```python
from build123d import *

# Parameters (mm, degrees)
SKETCH_1_W          = 45
SKETCH_1_H          = 4
SKETCH_1_W_2        = 5
EXTRUDE_1_DEPTH     = 84
SKETCH_2_W          = 20
SKETCH_2_H          = 20
CUT_EXTRUDE_1_DEPTH = 14
EXTRUDE_2_DEPTH     = 84


with BuildPart() as part:
    # Эскиз1 → Бобышка-Вытянуть1 (new body)
    with BuildSketch(Plane(origin=(0, 0, 0), x_dir=(0, 0, -1), z_dir=(1, 0, 0))):
        with Locations((22.5, 2)):
            Rectangle(SKETCH_1_W, SKETCH_1_H)
        with Locations((47.5, 2)):
            Rectangle(SKETCH_1_W_2, SKETCH_1_H)
        Polygon((45, 29), (45, 4), (50, 4), (50, 26.569712745), (48.596872999, 29), align=None)
        with Locations((22.5, 31)):
            Rectangle(SKETCH_1_W, SKETCH_1_H)
        Polygon((45, 33), (45, 29), (48.596872999, 29), (46.287471923, 33), align=None)
        Polygon((48.596872999, 29), (50, 26.569712745), (50, 29), align=None)
        Polygon((50, 29), (50, 26.569712745), (65.186719292, 0.265543331), (68.650820907, 2.265543331), (8.650820907, 106.188591785), (5.186719292, 104.188591785), (46.287471923, 33), (50, 33), align=None)
        Polygon((46.287471923, 33), (48.596872999, 29), (50, 29), (50, 33), align=None)
    extrude(amount=EXTRUDE_1_DEPTH)

    # Эскиз2 → Вырез-Вытянуть1 (cut)
    with BuildSketch(Plane.XZ):
        with Locations((74, -10)):
            Rectangle(SKETCH_2_W, SKETCH_2_H)
    extrude(amount=-CUT_EXTRUDE_1_DEPTH, mode=Mode.SUBTRACT)

    # Эскиз3 → Бобышка-Вытянуть2 (add)
    with BuildSketch(Plane(origin=(84, 0, 0), x_dir=(0, 0, -1), z_dir=(1, 0, 0))):
        Polygon((68.650820907, 2.265543331), (72.114922522, 4.265543331), (70.614922522, 6.863619543), (67.150820907, 4.863619543), align=None)
        Polygon((40.778226629, 42.54229276), (40.778226629, 33), (46.287471923, 33), align=None)
        Polygon((50, 26.569712745), (50, 18.552766001), (54.628586361, 18.552766001), align=None)
    extrude(amount=-EXTRUDE_2_DEPTH)


solid = part.part
```
The model under review builds one solid part; all positions refer to its coordinate system, in mm. A direction names the side the tool comes from. Coordinates: 2 decimals unless noted, no trailing zeros. Write each loop counter-clockwise with the first axis right and the second up, starting at its lowest first coordinate (ties: lowest second). Pieces come first, ordered by that corner, then holes. Notation, with made-up numbers: (7.25, 30) -> (58.25, 30) arc R19 cw to (58.25, 60) -> close; hole circle Ø5 at (82.25, 85). An arc over 180 degrees is marked (long way). One line per item, written item: value. Start each with the question number.
Q1. Add section D-D, the plane y = 27.5. Give the boundary of the cut face in (x, z).
Q2. The part is to be moulded in two halves that separate along Z. For faces 5 (the face through (42.6, 5.5, -71.4)), 6 (the face through (41, 9, -50)), 7 (the face through (64, 2, -10)), say which applies: +Z half, -Z half, draft (parallel to the pull), parting line (faces both ways), or undercut.
Q3. To check wall thickness, follow probe 1 along Y at (x, z) = (54, -4); probe 2 along Y at (x, z) = (61, -33); probe 3 along Y at (x, z) = (76, -23.5). State the ranges of each line that lie inside material, in increasing order.
Q4. Add section A-A, the plane z = -33. Give the boundary of the cut face in (x, y), then the cut area to 3 significant figures.
Q5. Clearance check with flat-ended pins moving along their axes: P1, Ø13.5, axis at x = 46.5, z = -28, coming from the +Y side; P2, Ø2.5, axis at x = 51, z = -52, coming from the -Y side; P3, Ø3, axis at x = 31.5, y = 55, coming from the -Z side; P4, Ø3, axis at x = 62.5, z = -16.5, coming from the -Y side. State where each tip first meets the part, or that it passes through.
Q6. Add section B-B, the plane x = 54. Give the boundary of the cut face in (y, z), then the cut area to 3 significant figures.
Q7. For faces 1 (the face through (74, 2, -20)), 2 (the face through (42.59, 5.88, -68.91)), 3 (the face through (41, 17, -45)), 4 (the face through (41.41, 9.54, -59.83)), list the 3-axis set-ups (+Z, -Z, +X, -X, +Y, -Y) from which the entire face can be reached by the end or side of a thin tool; tool diameter is ignored.
Q8. Add section C-C, the plane x = 67. Give the boundary of the cut face in (y, z), then the cut area to 3 significant figures.
Response:
1. outline: (0, -54.08) -> (84, -54.08) -> (84, -45) -> (0, -45) -> close
2. face 5: -Z half
2. face 6: undercut
2. face 7: draft
3. probe 1: 0 to 4, 29 to 33
3. probe 2: 0 to 4, 29 to 33, 56.01 to 64.01
3. probe 3: 0 to 4, 29 to 33, 72.47 to 80.47
4. outline: (0, 0) -> (84, 0) -> (84, 4) -> (0, 4) -> close; (0, 29) -> (84, 29) -> (84, 33) -> (0, 33) -> close; (0, 56.01) -> (84, 56.01) -> (84, 64.01) -> (0, 64.01) -> close
4. area: 1,340 mm²
5. P1: y = 84.37
5. P2: y = 18.55
5. P3: z = -39.07
5. P4: y = 0
6. outline: (0, -50) -> (18.55, -50) -> (18.55, -54.63) -> (0.27, -65.19) -> (4.27, -72.11) -> (6.86, -70.61) -> (4.86, -67.15) -> (106.19, -8.65) -> (104.19, -5.19) -> (42.54, -40.78) -> (33, -40.78) -> (33, 0) -> (29, 0) -> (29, -45) -> (4, -45) -> (4, 0) -> (0, 0) -> close
6. area: 1,050 mm²
7. face 1: +Z, +X, -Y
7. face 2: +X, -X, +Y
7. face 3: +Z, +X, -X
7. face 4: +X, -X, -Y
8. outline: (0, -50) -> (18.55, -50) -> (18.55, -54.63) -> (0.27, -65.19) -> (4.27, -72.11) -> (6.86, -70.61) -> (4.86, -67.15) -> (106.19, -8.65) -> (104.19, -5.19) -> (42.54, -40.78) -> (33, -40.78) -> (33, 0) -> (29, 0) -> (29, -45) -> (4, -45) -> (4, -20) -> (0, -20) -> close
8. area: 970 mm²
